Part model, mm, in its own coordinate system. Give positions to 0.01 mm unless a question says otherwise; leave off trailing zeros. Order: outer loops, then holes, each group sorted by start corner. A loop starts at its lowest first (then second) coordinate and runs counter-clockwise, first axis right, second up. Notation, with made-up numbers: (85, 57.5) - (138, 57.5) arc R25 ccw to (138, 73.5) - close; hole circle Ø2 at (-24.5, 24). An arc over 180 degrees is marked (long way). Use a Markdown table: item, result. Add a question column.
from build123d import *

# Parameters (mm, degrees)
SKETCH1_R           = 1.5
BOSS_EXTRUDE1_DEPTH = 3.175


with BuildPart() as part:
    # Sketch1 → Boss-Extrude1 (new body)
    with BuildSketch(Plane.XY):
        with BuildLine():
            Line((-8.73125, -69.500247016), (0, -69.500247016))
            Line((0, -69.500247016), (8.73125, -69.500247016))
            Line((8.73125, -69.500247016), (8.73125, -53.500247016))
            ThreePointArc((8.73125, -53.500247016), (0, -54.208035911), (-8.73125, -53.500247016))
            Line((-8.73125, -53.500247016), (-8.73125, -69.500247016))
        make_face()
        with Locations((-5.55625, -65.589370266)):
            Circle(SKETCH1_R, mode=Mode.SUBTRACT)
        with BuildLine():
            ThreePointArc((7.05625, -65.589370266), (5.55625, -67.089370266), (4.05625, -65.589370266))
            ThreePointArc((4.05625, -65.589370266), (5.55625, -64.089370266), (7.05625, -65.589370266))
        make_face(mode=Mode.SUBTRACT)
    extrude(amount=BOSS_EXTRUDE1_DEPTH)


solid = part.part
1. Cut at C-C (x = 5). Write the cut outline in (y, z) (3 decimals).
2. Pin check, flat tip, straight feed: P1, Ø1.8, axis at x = -5.56, y = -65.59, coming from the -Z side. Stop position of the tip, or through.
3. Drill centre lines: probe 1 along X at (y, z) = (-65.25, 0.2); probe 2 along Y at (x, z) = (4.25, 1.55); probe 3 along Y at (x, z) = (-5.5, 0.75). Where is each one in solid material? Low to high. Write a range as [from, to].
4. Cut at D-D (x = 1.5). Write the cut outline in (y, z) (3 decimals).
5. Mould opens along Y. For faces 1 (the face through (0, -61, 0)), 2 (the face through (-4.75, -64.325, 1.565)), 3 (the face through (0.123, -54.208, 1.565)), 4 (the face through (4.75, -64.325, 1.565)) say: released by +Y, released by -Y, zero draft, split by the parting line, or undercut.
6. Cut at B-B (z = 0.7). Write the cut outline in (x, y), plus the area to 3 significant figures.
7. Cut at A-A (x = -6.25). Write the cut outline in (y, z) (3 decimals).
Responses:
| question | item | result |
|---|---|---|
| 1 | outline | (-69.5, 0) - (-66.982, 0) - (-66.982, 3.175) - (-69.5, 3.175) - close; (-64.196, 0) - (-53.977, 0) - (-53.977, 3.175) - (-64.196, 3.175) - close |
| 2 | P1 | passes through |
| 3 | probe 1 | x = [-8.73, -7.02], [-4.1, 4.1], [7.02, 8.73] |
| 3 | probe 2 | y = [-69.5, -66.33], [-64.85, -54.04] |
| 3 | probe 3 | y = [-69.5, -67.09], [-64.09, -53.93] |
| 4 | outline | (-69.5, 0) - (-54.187, 0) - (-54.187, 3.175) - (-69.5, 3.175) - close |
| 5 | face 1 | zero draft |
| 5 | face 2 | undercut |
| 5 | face 3 | released by +Y |
| 5 | face 4 | undercut |
| 6 | outline | (-8.73, -69.5) - (8.73, -69.5) - (8.73, -53.5) arc R54.21 cw to (-8.73, -53.5) - close; hole circle Ø3 at (-5.56, -65.59); hole circle Ø3 at (5.56, -65.59) |
| 6 | area | 257 mm² |
| 7 | outline | (-69.5, 0) - (-66.919, 0) - (-66.919, 3.175) - (-69.5, 3.175) - close; (-64.259, 0) - (-53.847, 0) - (-53.847, 3.175) - (-64.259, 3.175) - close |
